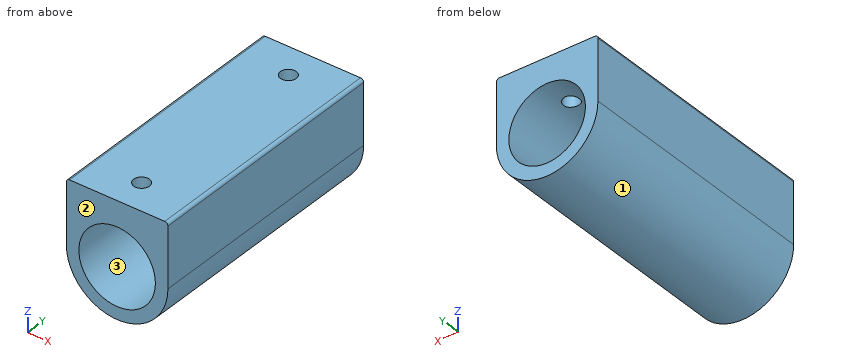
from build123d import *

# Parameters (mm, degrees)
F0_R     = 6.025
F1_DEPTH = 40
F2_R     = 1.25
F3_DEPTH = 4.1
F4_R     = 0.5


with BuildPart() as f1:
    # F0 (on Front) → F1 (new body)
    with BuildSketch(Plane.XZ):
        with BuildLine():
            Line((-8, 10), (-8, 0))
            ThreePointArc((-8, 0), (0, -8), (8, 0))
            Line((8, 0), (8, 10))
            Line((8, 10), (-8, 10))
        make_face()
        Circle(F0_R, mode=Mode.SUBTRACT)
    extrude(amount=F1_DEPTH)

    # F2 (on face) → F3 (cut)
    with BuildSketch(Plane.XY.offset(10)):
        with Locations((0, -5)):
            Circle(F2_R)
        with Locations((0, -35)):
            Circle(F2_R)
    extrude(amount=-F3_DEPTH, mode=Mode.SUBTRACT)

    # F4
    f4_edges = [f1.edges().sort_by_distance(p)[0] for p in [
        (-8, -20, 10),
        (8, -20, 10),
    ]]
    fillet(f4_edges, radius=F4_R)


solid = f1.part
Geometry check sheet. Reference: the model listing, model coordinates, mm. Face numbers are marked on the shaded views. Give positions to 0.01 mm unless a question says otherwise; leave off trailing zeros. Write each loop counter-clockwise with the first axis right and the second up, starting at its lowest first coordinate (ties: lowest second). Pieces come first, ordered by that corner, then holes.
1) Cross-section at D-D (x = -5.5). Record the boundary of the cut face in (y, z).
Values follow:
outline: (-40, -5.81) - (0, -5.81) - (0, -2.46) - (-40, -2.46) - close; (-40, 2.46) - (0, 2.46) - (0, 10) - (-40, 10) - close
2) Cross-section at A-A (x = 0). Record the boundary of the cut face in (y, z) (3 decimals), plus the area to 3 significant figures.
Values follow:
outline: (-40, -8) - (0, -8) - (0, -6.025) - (-40, -6.025) - close; (-40, 6.025) - (-36.25, 6.025) - (-36.25, 10) - (-40, 10) - close; (-33.75, 6.025) - (-6.25, 6.025) - (-6.25, 10) - (-33.75, 10) - close; (-3.75, 6.025) - (0, 6.025) - (0, 10) - (-3.75, 10) - close
area: 218 mm2
3) Release check for a two-part mould opening along Z. For the marked faces 1, 2 and 3 record: released by +Z, released by -Z, zero draft, split by the parting line, or undercut.
Values follow:
face 1: released by -Z
face 2: zero draft
face 3: undercut
4) Cross-section at C-C (z = 2.5). Record the boundary of the cut face in (x, y), plus the area to 3 significant figures.
Values follow:
outline: (-8, -40) - (-5.48, -40) - (-5.48, 0) - (-8, 0) - close; (5.48, -40) - (8, -40) - (8, 0) - (5.48, 0) - close
area: 201 mm2
5) Cross-section at B-B (y = -3). Record the boundary of the cut face in (x, z) (3 decimals), plus the area to 3 significant figures.
Values follow:
outline: (-8, 0) arc R8 ccw to (8, 0) - (8, 9.5) arc R0.5 ccw to (7.5, 10) - (-7.5, 10) arc R0.5 ccw to (-8, 9.5) - close; hole circle Ø12.05 at (0, 0)
area: 146 mm2
6) Go/stop test with flat-tipped pins: pin 1 Ø8 at (y, z) = (-28, -4) entering from +X; pin 2 Ø3 at (y, z) = (-8, -2) entering from -X. Record where each tip stops, or that it passes through.
Values follow:
pin 1: stops at x = 8
pin 2: stops at x = -7.98
7) Thickness scan on line 1 (Y direction, x = 0, z = 7.2); line 2 (Y direction, x = 1, z = 6); line 3 (X direction, y = -5, z = 8.55). Record the ranges inside material, lowest first.
Values follow:
line 1: y = -40 to -36.25, -33.75 to -6.25, -3.75 to 0
line 2: y = -40 to -35.75, -34.25 to -5.75, -4.25 to 0
line 3: x = -8 to -1.25, 1.25 to 8
